Model file for the job. Use its own axes, mm. Face numbers are marked on the shaded views. Round coordinates to 2 decimals unless told otherwise and drop trailing zeros. Loops run counter-clockwise (first coordinate to the right, second up) from the corner with the lowest first, then second, coordinate; pieces in that order, holes last. Notation, with made-up numbers: M 40,32.25 L 80,32.25 A30 cw 80,70.25 Z; hole C 9,79 d5. An arc over 180 degrees is marked long. Answer in a Markdown table with one row per item.
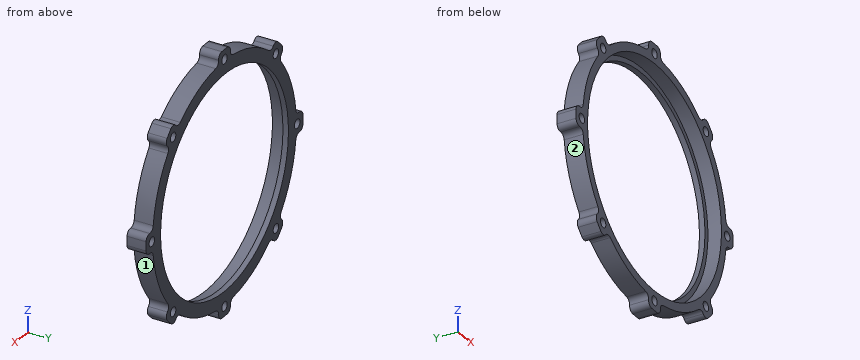
from build123d import *

# Parameters (mm, degrees)
PATTERN_CIRCULAR_1_COUNT = 8
CUT_EXTRUDE_START        = -10
CUT_EXTRUDE_1_DEPTH      = 10
PATTERN_CIRCULAR_2_COUNT = 8
FILLET_2_R               = 2


with BuildPart() as part:
    # 草图1 → 旋转1 (revolve)
    with BuildSketch(Plane.XY, mode=Mode.PRIVATE) as revolve_1_sk:
        Polygon((-40.5, 0), (-47.5, 0), (-47.5, 6.9), (-38.7, 6.9), (-38.7, 4.9), (-40.5, 4.9), align=None)
    revolve(revolve_1_sk.sketch.rotate(Axis((0, 0, 0), (0, 1, 0)), 270), axis=Axis((0, 0, 0), (0, 1, 0)))

    # 草图4 → M4 螺纹孔1 (revolve, cut)
    with BuildSketch(Plane(origin=(0, 0, 44), x_dir=(0, 0, -1), z_dir=(1, 0, 0))):
        Polygon((0, 0), (0, 8.991420021), (1.65, 8), (1.65, 0), align=None)
    hole_wizard_m4_1 = revolve(axis=Axis((0, -6.35, 44), (0, 1, 0)), mode=Mode.SUBTRACT)

    # 阵列(圆周)1: M4 螺纹孔1 ×8 about axis
    pattern_circular_1_axis = Axis((0, 0, 0), (0, 1, 0))
    for i in range(1, PATTERN_CIRCULAR_1_COUNT):
        add(hole_wizard_m4_1.rotate(pattern_circular_1_axis, i * 360 / PATTERN_CIRCULAR_1_COUNT), mode=Mode.SUBTRACT)

    # 草图5 → 切除-拉伸1 (cut)
    with BuildSketch(Plane.XZ.offset(CUT_EXTRUDE_START)):
        with BuildLine():
            Line((-30.848782296, 36.119283366), (-28.250990102, 33.077659504))
            ThreePointArc((-28.250990102, 33.077659504), (-16.646729308, 40.188759664), (-3.412970664, 43.365904017))
            Line((-3.412970664, 43.365904017), (-3.726807047, 47.353573352))
            ThreePointArc((-3.726807047, 47.353573352), (-18.177463037, 43.884277794), (-30.848782296, 36.119283366))
        make_face()
    cut_extrude_1 = extrude(amount=CUT_EXTRUDE_1_DEPTH, mode=Mode.SUBTRACT)

    # 阵列(圆周)2: 切除-拉伸1 ×8 about axis
    pattern_circular_2_axis = Axis((0, 0, 0), (0, 1, 0))
    for i in range(1, PATTERN_CIRCULAR_2_COUNT):
        add(cut_extrude_1.rotate(pattern_circular_2_axis, i * 360 / PATTERN_CIRCULAR_2_COUNT), mode=Mode.SUBTRACT)

    # 圆角2
    fillet_2_edges = [part.edges().sort_by_distance(p)[0] for p in [
        (-3.412970664, 3.45, 43.365904017),
        (-28.250990102, 3.45, 33.077659504),
        (-30.848782296, 3.45, 36.119283366),
        (-36.119283366, 3.45, 30.848782296),
        (-33.077659504, 3.45, 28.250990102),
        (-43.365904017, 3.45, 3.412970664),
        (-47.353573352, 3.45, 3.726807047),
        (-47.353573352, 3.45, -3.726807047),
        (-43.365904017, 3.45, -3.412970664),
        (-33.077659504, 3.45, -28.250990102),
        (-36.119283366, 3.45, -30.848782296),
        (-30.848782296, 3.45, -36.119283366),
        (-28.250990102, 3.45, -33.077659504),
        (-3.412970664, 3.45, -43.365904017),
        (-3.726807047, 3.45, -47.353573352),
        (3.726807047, 3.45, -47.353573352),
        (3.412970664, 3.45, -43.365904017),
        (28.250990102, 3.45, -33.077659504),
        (30.848782296, 3.45, -36.119283366),
        (36.119283366, 3.45, -30.848782296),
        (33.077659504, 3.45, -28.250990102),
        (43.365904017, 3.45, -3.412970664),
        (47.353573352, 3.45, -3.726807047),
        (47.353573352, 3.45, 3.726807047),
        (43.365904017, 3.45, 3.412970664),
        (33.077659504, 3.45, 28.250990102),
        (36.119283366, 3.45, 30.848782296),
        (30.848782296, 3.45, 36.119283366),
        (28.250990102, 3.45, 33.077659504),
        (3.412970664, 3.45, 43.365904017),
        (3.726807047, 3.45, 47.353573352),
        (-3.726807047, 3.45, 47.353573352),
    ]]
    fillet(fillet_2_edges, radius=FILLET_2_R - 0.0001)  # a hair under: the kernel refuses the full size


solid = part.part
1. Mould opens along X. For the marked faces 1 and 2 say: +X half, -X half, draft (parallel to the pull), parting line (faces both ways), or undercut.
Verdict:
| item | result |
|---|---|
| face 1 | +X half |
| face 2 | -X half |
2. Saw through at C-C (z = -20.5). Write the cut outline in (x, y).
Verdict:
| item | result |
|---|---|
| outline | M -38.37,0 L -34.93,0 L -34.93,4.9 L -32.82,4.9 L -32.82,6.9 L -38.37,6.9 Z; M 32.82,4.9 L 34.93,4.9 L 34.93,0 L 38.37,0 L 38.37,6.9 L 32.82,6.9 Z |
3. Wall check: probe 1 along Z at (x, y) = (0.5, 1.5); probe 2 along X at (y, z) = (1, 1); probe 3 along X at (y, z) = (3, 16.5). Give the ranges that are in metal, low to high.
Verdict:
| item | result |
|---|---|
| probe 1 | z = -47.5 to -45.57, -42.43 to -40.5, 40.5 to 42.43, 45.57 to 47.5 |
| probe 2 | x = -47.49 to -45.31, -42.69 to -40.49, 40.49 to 42.69, 45.31 to 47.49 |
| probe 3 | x = -40.25 to -36.99, 36.99 to 40.25 |
4. Saw through at D-D (x = -37.5). Write the cut outline in (y, z).
Verdict:
| item | result |
|---|---|
| outline | M 0,-22.05 L 6.9,-22.05 L 6.9,-9.56 L 4.9,-9.56 L 4.9,-15.3 L 0,-15.3 Z; M 0,15.3 L 4.9,15.3 L 4.9,9.56 L 6.9,9.56 L 6.9,22.05 L 0,22.05 Z |
5. Pin check, flat tips, straight feed: pin 1 (1 mm diameter, centred on y = 4.5, z = -17.5, fed in from +X); pin 2 (1.5 mm diameter, centred on x = -27, y = 1, fed in from -Z); pin 3 (3 mm diameter, centred on y = 3.5, z = 12, fed in from +X). Stop position of each tip, or through.
Verdict:
| item | result |
|---|---|
| pin 1 | stops at x = 40.04 |
| pin 2 | stops at z = -34.69 |
| pin 3 | stops at x = 42.21 |
6. Saw through at A-A (z = 0). Write the cut outline in (x, y).
Verdict:
| item | result |
|---|---|
| outline | M -47.5,0 L -45.65,0 L -45.65,6.9 L -47.5,6.9 Z; M -42.35,0 L -40.5,0 L -40.5,4.9 L -38.7,4.9 L -38.7,6.9 L -42.35,6.9 Z; M 38.7,4.9 L 40.5,4.9 L 40.5,0 L 42.35,0 L 42.35,6.9 L 38.7,6.9 Z; M 45.65,0 L 47.5,0 L 47.5,6.9 L 45.65,6.9 Z |
7. Saw through at B-B (x = 0). Write the cut outline in (y, z), and give its area (3 significant figures).
Verdict:
| item | result |
|---|---|
| outline | M 0,-47.5 L 6.9,-47.5 L 6.9,-45.65 L 0,-45.65 Z; M 0,-42.35 L 6.9,-42.35 L 6.9,-38.7 L 4.9,-38.7 L 4.9,-40.5 L 0,-40.5 Z; M 0,40.5 L 4.9,40.5 L 4.9,38.7 L 6.9,38.7 L 6.9,42.35 L 0,42.35 Z; M 0,45.65 L 6.9,45.65 L 6.9,47.5 L 0,47.5 Z |
| area | 58.3 mm² |
